Autodesk Inventor part; units mm, degrees
ref_plane "Work Plane1" through (0, -29, 0) normal (0, 0, 1) x (1, 0, 0)
ref_plane "YZ Plane" through (0, 0, 0) normal (1, 0, 0) x (0, 1, 0)
ref_plane "XZ Plane" through (0, 0, 0) normal (0, 1, 0) x (-1, 0, 0)
sketch "Sketch1" plane through (0, 0, 0) normal (1, 0, 0) x (0, 1, 0)
  line L0 (29, 22) -> (-29, 22)
  line L1 (-29, 22) -> (-29, -22)
  line L2 (-29, -22) -> (29, -22)
  line L3 (29, -22) -> (29, 22)
  dimension "d4" = 58
  dimension "d5" = 44
extrude "Extrusion1" add sketch "Sketch1" along normal blind 82.5
sketch "Sketch2" plane through (82.5, 0, 0) normal (1, 0, 0) x (0, 0, -1)
  circle A0 centre (0, 0) radius 22
  dimension "d8" = 44
extrude "Extrusion2" add sketch "Sketch2" along normal blind 60
sketch "Sketch3" plane through (142.5, 0, 0) normal (1, 0, 0) x (0, 0, -1)
  circle A0 centre (0, 0) radius 20
  dimension "d11" = 40
extrude "Extrusion3" add sketch "Sketch3" along normal blind 4
sketch "Sketch4" plane through (146.5, 0, 0) normal (1, 0, 0) x (0, 0, -1)
  circle A0 centre (0, 0) radius 19
  dimension "d14" = 38
extrude "Extrusion4" add sketch "Sketch4" along normal blind 2
sketch "Sketch5" plane through (148.5, 0, 0) normal (1, 0, 0) x (0, 0, -1)
  circle A0 centre (0, 0) radius 10
  dimension "d17" = 20
extrude "Extrusion5" add sketch "Sketch5" along normal blind 2
sketch "Sketch6" plane through (0, -29, -22) normal (0, 0, -1) x (-1, 0, 0)
  circle A0 centre (-25, 29) radius 12.5
  point P0 (0, 29)
  dimension "d21" = 25
extrude "Extrusion6" add sketch "Sketch6" along normal blind 5
sketch "Sketch7" plane through (0, -29, -22) normal (0, 0, -1) x (-1, 0, 0)
  line L0 (0, 0) -> (-82.5, 0)
  line L1 (0, 0) -> (0, 58)
  circle A0 centre (-13, 10) radius 5
  line L2 (-82.5, 29) -> (-82.5, 58)
  circle A1 centre (-13, 48) radius 5
  point P0 (0, 29)
  dimension "d28" = 10
extrude "Extrusion7" add sketch "Sketch7" along normal blind 2.5
sketch "Sketch8" plane through (0, -29, -22) normal (0, 0, -1) x (-1, 0, 0)
  line L0 (0, 0) -> (-82.5, 0)
  circle A0 centre (-55, 10) radius 5
  point P0 (0, 29)
  dimension "d33" = 10
extrude "Extrusion8" add sketch "Sketch8" along normal blind 2.5
sketch "Sketch9" plane through (0, -29, -22) normal (0, 0, -1) x (-1, 0, 0)
  circle A0 centre (-69, 48) radius 5
  point P0 (0, 29)
  point P1 (0, 58)
  dimension "d38" = 10
extrude "Extrusion9" add sketch "Sketch9" along normal blind 2.5
sketch "Sketch10" plane through (55, -19, -24.5) normal (0, 0, -1) x (-1, 0, 0)
  circle A0 centre (0, 0) radius 2
  point P0 (55, 19)
  dimension "d41" = 4
extrude "Extrusion10" cut sketch "Sketch10" against normal blind 5
sketch "Sketch11" plane through (69, 19, -24.5) normal (0, 0, -1) x (-1, 0, 0)
  circle A0 centre (0, 0) radius 2
  point P0 (69, -19)
  dimension "d44" = 4
extrude "Extrusion11" cut sketch "Sketch11" against normal blind 4
sketch "Sketch12" plane through (13, -19, -24.5) normal (0, 0, -1) x (-1, 0, 0)
  circle A0 centre (0, 0) radius 2
  point P0 (13, 19)
  dimension "d47" = 4
extrude "Extrusion12" cut sketch "Sketch12" against normal blind 4
sketch "Sketch13" plane through (13, 19, -24.5) normal (0, 0, -1) x (-1, 0, 0)
  circle A0 centre (0, 0) radius 2
  point P0 (13, -19)
  dimension "d50" = 4
extrude "Extrusion13" cut sketch "Sketch13" against normal blind 4
sketch "Sketch14" plane through (25, 0, -27) normal (0, 0, -1) x (-1, 0, 0)
  circle A0 centre (0, 0) radius 5
  point P0 (25, 0)
  dimension "d53" = 10
extrude "Extrusion14" add sketch "Sketch14" along normal blind 9
sketch "Sketch15" plane through (25, 0, -36) normal (0, 0, -1) x (-1, 0, 0)
  circle A0 centre (0, 0) radius 5
  line L0 (3.5, -3.5707) -> (3.5, 3.5707)
  arc A1 (3.5, 3.5707) -> (3.5, -3.5707) centre (0, 0) ccw
  point P0 (25, 0)
extrude "Extrusion15" add sketch "Sketch15" along normal blind 15 contours L0 A0 picked at (0.6794, -0.2053)
ref_plane "Work Plane1" through (0, -29, 0) normal (0, 0, 1) x (1, 0, 0)
mirror "Mirror1" about plane through (0, -29, 0) normal (0, 0, 1) of "Extrusion8", "Extrusion10", "Extrusion9", "Extrusion11", "Extrusion6", "Extrusion14", "Extrusion15", "Extrusion7", "Extrusion12", "Extrusion13"
equation "\"d45\" = d44"
equation "\"d48\" = d47"
equation "\"d51\" = d50"
properties part number "GEARBOX PURNIMA SAMARARATNE" material "Steel"
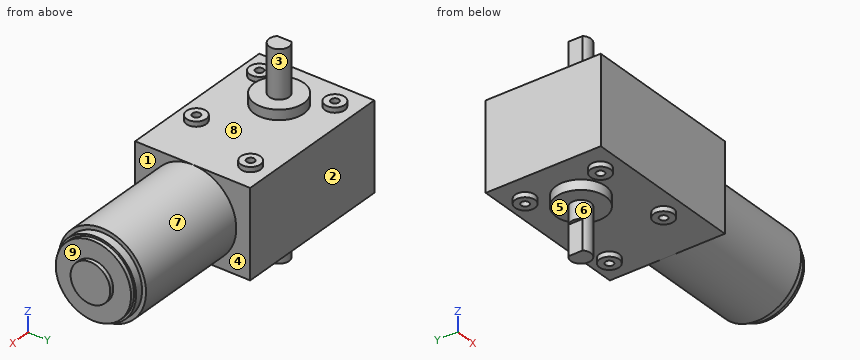
Geometry: final body of the model. Coordinates: model frame, mm. Face numbers are marked on the shaded views. A direction names the side the tool comes from. Coordinates: 2 decimals unless noted, no trailing zeros. Order: outer loops, then holes, each group sorted by start corner. A loop starts at its lowest first (then second) coordinate and runs counter-clockwise, first axis right, second up.
Item 1: Contact query for flat-ended pins moving along their axis: P1, Ø8, axis at y = 1, z = -41.5, coming from the -X side; P2, Ø11, axis at x = 12.5, y = 19.5, coming from the +Z side; P3, Ø12, axis at x = 96.5, z = 9, coming from the +Y side. Output: stop coordinate, or through.
Answer:
P1: stops at x = 21.5
P2: stops at z = 24.5
P3: stops at y = 21.79
Item 2: Section query A-A (x = 25). Output: boundary loops of the cut face in (y, z).
Answer:
outline: (-29, -22) - (-12.5, -22) - (-12.5, -27) - (-5, -27) - (-5, -51) - (5, -51) - (5, -27) - (12.5, -27) - (12.5, -22) - (29, -22) - (29, 22) - (12.5, 22) - (12.5, 27) - (5, 27) - (5, 51) - (-5, 51) - (-5, 27) - (-12.5, 27) - (-12.5, 22) - (-29, 22) - close
Item 3: Access query for the marked faces 1, 2, 3, 4 and 5. Directions: +Z, -Z, +X, -X, +Y, -Y. A direction counts if a zero-diameter tool reaches every point of the face in a straight line with its end or side. Return the directions, or none.
Answer:
face 1: +X, -Y
face 2: +Z, -Z, +X, -X, +Y
face 3: +Z
face 4: +X, +Y
face 5: -Z
Item 4: Section query C-C (z = -16). Output: boundary loops of the cut face in (x, y).
Answer:
outline: (0, -29) - (82.5, -29) - (82.5, -15.1) - (142.5, -15.1) - (142.5, -12) - (146.5, -12) - (146.5, -10.25) - (148.5, -10.25) - (148.5, 10.25) - (146.5, 10.25) - (146.5, 12) - (142.5, 12) - (142.5, 15.1) - (82.5, 15.1) - (82.5, 29) - (0, 29) - close
Item 5: Section query B-B (z = 0). Output: boundary loops of the cut face in (x, y), then the cut area to 3 significant figures.
Answer:
outline: (0, -29) - (82.5, -29) - (82.5, -22) - (142.5, -22) - (142.5, -20) - (146.5, -20) - (146.5, -19) - (148.5, -19) - (148.5, -10) - (150.5, -10) - (150.5, 10) - (148.5, 10) - (148.5, 19) - (146.5, 19) - (146.5, 20) - (142.5, 20) - (142.5, 22) - (82.5, 22) - (82.5, 29) - (0, 29) - close
area: 7,700 mm2
Item 6: Material intervals for line 1 along Y through (x, z) = (55, -23); line 2 along Z through (x, y) = (44.5, 26); line 3 along X through (y, z) = (11, -18.5), sorted ascending.
Answer:
line 1: y = -24 to -21, -17 to -14
line 2: z = -22 to 22
line 3: x = 0 to 142.5
Item 7: Section query D-D (x = 41). Output: boundary loops of the cut face in (y, z).
Answer:
outline: (-29, -22) - (29, -22) - (29, 22) - (-29, 22) - close
Item 8: Draft query along X for the marked faces 6, 7, 8 and 9. Return one class per face: released by +X, released by -X, zero draft, split by the parting line, or undercut.
Answer:
face 6: split by the parting line
face 7: zero draft
face 8: undercut
face 9: released by +X
